```python
from build123d import *

# Parameters (mm, degrees)
F1_DEPTH  = 0.5
F2_W      = 2.5
F2_H      = 5
F3_DEPTH  = 0.501
F4_DEPTH  = 1
F6_DEPTH  = 0.5
F8_DEPTH  = 0.1
F10_DEPTH = 0.25


# Not quite as in the source:
# - a feature names something its author has since deleted; it is built from what else it names


with BuildPart() as f1:
    # F0 (on Top) → F1 (new body)
    with BuildSketch(Plane.XY):
        with BuildLine():
            Line((0, 4.5), (-13.5, 4.5))
            ThreePointArc((-13.5, 4.5), (-18, 0), (-13.5, -4.5))
            Line((-13.5, -4.5), (0, -4.5))
            Line((0, -4.5), (13.5, -4.5))
            ThreePointArc((13.5, -4.5), (18, 0), (13.5, 4.5))
            Line((13.5, 4.5), (0, 4.5))
        make_face()
    extrude(amount=F1_DEPTH)

    # F2 (on face) → F3 (cut, through all)
    with BuildSketch(Plane.XY.offset(0.5)):
        with Locations((-12.25, 0)):
            Rectangle(F2_W, F2_H)
        with Locations((-5.25, 0)):
            Rectangle(F2_W, F2_H)
        with Locations((-1.75, 0)):
            Rectangle(F2_W, F2_H)
        with Locations((-8.75, 0)):
            Rectangle(F2_W, F2_H)
        with Locations((1.75, 0)):
            Rectangle(F2_W, F2_H)
        with Locations((5.25, 0)):
            Rectangle(F2_W, F2_H)
        with Locations((8.75, 0)):
            Rectangle(F2_W, F2_H)
        with Locations((12.25, 0)):
            Rectangle(F2_W, F2_H)
    extrude(amount=-F3_DEPTH, mode=Mode.SUBTRACT)

    # F2 (on face) → F4 (join)
    with BuildSketch(Plane.XY.offset(0.5)):
        with BuildLine():
            Line((0, 4.5), (-13.5, 4.5))
            ThreePointArc((-13.5, 4.5), (-18, 0), (-13.5, -4.5))
            Line((-13.5, -4.5), (0, -4.5))
            Line((0, -4.5), (13.5, -4.5))
            ThreePointArc((13.5, -4.5), (18, 0), (13.5, 4.5))
            Line((13.5, 4.5), (0, 4.5))
        make_face()
        with BuildLine():
            ThreePointArc((-13.5, -3.5), (-17, 0), (-13.5, 3.5))
            Line((-13.5, 3.5), (0, 3.5))
            Line((0, 3.5), (13.5, 3.5))
            ThreePointArc((13.5, 3.5), (17, 0), (13.5, -3.5))
            Line((13.5, -3.5), (0, -3.5))
            Line((0, -3.5), (-13.5, -3.5))
        make_face(mode=Mode.SUBTRACT)
    extrude(amount=F4_DEPTH)

    # F5 (on face) → F6 (join)
    with BuildSketch(Plane.XY.offset(1.5)):
        with BuildLine():
            Line((0, 4.5), (-13.5, 4.5))
            ThreePointArc((-13.5, 4.5), (-18, 0), (-13.5, -4.5))
            Line((-13.5, -4.5), (0, -4.5))
            Line((0, -4.5), (13.5, -4.5))
            ThreePointArc((13.5, -4.5), (18, 0), (13.5, 4.5))
            Line((13.5, 4.5), (0, 4.5))
        make_face()
        with BuildLine():
            Line((13.5, -3.5), (-13.5, -3.5))
            ThreePointArc((-13.5, -3.5), (-17, 0), (-13.5, 3.5))
            Line((-13.5, 3.5), (13.5, 3.5))
            ThreePointArc((13.5, 3.5), (17, 0), (13.5, -3.5))
        make_face(mode=Mode.SUBTRACT)
        with BuildLine():
            ThreePointArc((-13.5, 3.5), (-17, 0), (-13.5, -3.5))
            Line((-13.5, -3.5), (13.5, -3.5))
            ThreePointArc((13.5, -3.5), (17, 0), (13.5, 3.5))
            Line((13.5, 3.5), (-13.5, 3.5))
        make_face()
        with BuildLine():
            ThreePointArc((-13.5, -2.5), (-16, 0), (-13.5, 2.5))
            Line((-13.5, 2.5), (0, 2.5))
            Line((0, 2.5), (13.5, 2.5))
            ThreePointArc((13.5, 2.5), (16, 0), (13.5, -2.5))
            Line((13.5, -2.5), (0, -2.5))
            Line((0, -2.5), (-13.5, -2.5))
        make_face(mode=Mode.SUBTRACT)
    extrude(amount=F6_DEPTH)

    # F7 (on face) → F8 (cut)
    with BuildSketch(Plane.XY.offset(0.5)):
        with BuildLine():
            ThreePointArc((-15.75, 0), (-15.25, -0.5), (-14.75, 0))
            ThreePointArc((-14.75, 0), (-15.25, 0.5), (-15.75, 0))
        make_face()
    extrude(amount=-F8_DEPTH, mode=Mode.SUBTRACT)

    # F9 (on face) → F10 (cut)
    with BuildSketch(Plane(origin=(0, 0, 0), x_dir=(1, 0, 0), z_dir=(0, 0, -1))):
        with BuildLine():
            ThreePointArc((-15.75, 0), (-15.25, -0.5), (-14.75, 0))
            ThreePointArc((-14.75, 0), (-15.25, 0.5), (-15.75, 0))
        make_face()
    extrude(amount=-F10_DEPTH, mode=Mode.SUBTRACT)


solid = f1.part
```
Geometry: final body of the model. Coordinates: model frame, mm. A direction names the side the tool comes from. Round coordinates to 2 decimals unless told otherwise and drop trailing zeros. Order: outer loops, then holes, each group sorted by start corner. A loop starts at its lowest first (then second) coordinate and runs counter-clockwise, first axis right, second up. Notation, with made-up numbers: (12, 3.5) - (23, 3.5) arc R21 ccw to (23, 39.5) - close; hole circle Ø2 at (17.25, -30). An arc over 180 degrees is marked (long way). Write item = value, one per line. Start each with the question number.
Q1. Cut plane A-A on x = -5. Return the cut outline in (y, z), and give its area (3 significant figures).
Q2. Cut plane B-B on y = 0. Give the number of separate pieces and of enclosed holes in the cut face, and give its area (4 significant figures).
Q3. Access query for faces 4 (the flat face through (0, -4.5, 1)), 5 (the flat face through (-15, 0, 0.25)), 6 (the cylindrical face through (17, 0, 1)), 7 (the cylindrical face through (16, 0.1, 1.7)), 8 (the flat face through (0, 0, 0)). Directions: +Z, -Z, +X, -X, +Y, -Y. A direction counts if a zero-diameter tool reaches every point of the face in a straight line with its end or side. Return the directions, or none.
Q4. Cut plane C-C on x = 14. Return the cut outline in (y, z).
Q5. Ray query, line 1 (Y direction, x = -9, z = 1.35); line 2 (Y direction, x = -3, z = 1.65); line 3 (Z direction, x = -2, y = -3.25). Return the intervals inside material, ascending. Write a range as from..to.
Q6. Pull-direction query (X, two-part tool) for faces 1 (the flat face through (0, -3, 2)), 2 (the flat face through (0, 3.5, 1)), 3 (the cylindrical face through (-18, 0, 1)); classes: +X half, -X half, draft (parallel to the pull), parting line (faces both ways), or undercut.
Outcome:
q1.outline = (-4.5, 0) - (-2.5, 0) - (-2.5, 0.5) - (-3.5, 0.5) - (-3.5, 1.5) - (-2.5, 1.5) - (-2.5, 2) - (-4.5, 2) - close; (2.5, 0) - (4.5, 0) - (4.5, 2) - (2.5, 2) - (2.5, 1.5) - (3.5, 1.5) - (3.5, 0.5) - (2.5, 0.5) - close
q1.area = 6.00 mm^2
q2.separate_pieces = 9
q2.enclosed_holes = 0
q2.area = 11.65 mm^2
q3.face_4 = +Z, -Z, +X, -X, -Y
q3.face_5 = -Z
q3.face_6 = none
q3.face_7 = +Z
q3.face_8 = -Z, +X, -X, +Y, -Y
q4.outline = (-4.47, 0) - (4.47, 0) - (4.47, 2) - (2.45, 2) - (2.45, 1.5) - (3.46, 1.5) - (3.46, 0.5) - (-3.46, 0.5) - (-3.46, 1.5) - (-2.45, 1.5) - (-2.45, 2) - (-4.47, 2) - close
q5.line_1 = -4.5..-3.5, 3.5..4.5
q5.line_2 = -4.5..-2.5, 2.5..4.5
q5.line_3 = 0..0.5, 1.5..2
q6.face_1 = draft
q6.face_2 = undercut
q6.face_3 = -X half
